Autodesk Inventor part; units mm, degrees
ref_plane "YZ Plane" through (0, 0, 0) normal (1, 0, 0) x (0, 1, 0)
ref_plane "XZ Plane" through (0, 0, 0) normal (0, 1, 0) x (-1, 0, 0)
ref_plane "XY Plane" through (0, 0, 0) normal (0, 0, 1) x (1, 0, 0)
sketch "Sketch1" plane through (0, 0, 0) normal (0, 1, 0) x (-1, 0, 0)
  line L0 (0, 0) -> (0, -167)
  circle A0 centre (0, 0) radius 1.7
  circle A1 centre (0, -167) radius 1.7
  circle A2 centre (0, 0) radius 2.5
  circle A3 centre (0, -167) radius 2.5
  line L1 (2.5, -167) -> (2.5, 0)
  line L2 (-2.5, 0) -> (-2.5, -167)
  dimension "d0" = 167
  dimension "d1" = 3.4
  dimension "d2" = 3.4
  dimension "d3" = 5
  dimension "d4" = 5
extrude "Extrusion1" add sketch "Sketch1" along normal blind 3
properties part number "HENK"
Check sheet for the modelled part. Datum: model origin and axes. Units: mm. Round coordinates to 2 decimals unless told otherwise and drop trailing zeros. Write each loop counter-clockwise with the first axis right and the second up, starting at its lowest first coordinate (ties: lowest second). Pieces come first, ordered by that corner, then holes. Notation, with made-up numbers: (-19, 43) -> (18, 43) arc R21 ccw to (18, 60) -> close; hole circle Ø11 at (-5.75, -19). An arc over 180 degrees is marked (long way). Answer as CSV lines item,"result". Start each with the question number.
1) Go/stop test with flat-tipped pins: P1, Ø1.5, axis at x = 1, y = 2, coming from the -Z side; P2, Ø2, axis at x = -1, z = -49, coming from the -Y side. Record where each tip stops, or that it passes through.
2) Material ranges on line 1 (Z direction, x = 0, y = 0.75); line 2 (X direction, y = 1.1, z = 0); line 3 (Z direction, x = 1.5, y = 1.3), recorded low to high. Write a range as from..to.
3) Release check for a two-part mould opening along Z. For faces 1 (the cylindrical face through (-0.1, 1.5, -169.5)), 2 (the cylindrical face through (0.37, 1.48, -165.34)), 3 (the flat face through (-2.5, 1, -85)), 4 (the cylindrical face through (0.1, 1.5, 2.5)) record: pulls with the +Z half, pulls with the -Z half, needs draft (parallel to the pull), parting line crosses it, or undercut.
4) Section check B-B on y = 2.1. Enter the section's corners in (x, z).
5) Section check A-A on x = 0. Enter the section's corners in (y, z).
Found:
1,P1,"stops at z = -169.49"
1,P2,"stops at y = 0"
2,line 1,"z = -169.5..-168.7, -165.3..-1.7, 1.7..2.5"
2,line 2,"x = -2.5..-1.7, 1.7..2.5"
2,line 3,"z = -169..-167.8, -166.2..-0.8, 0.8..2"
3,face 1,"pulls with the -Z half"
3,face 2,"undercut"
3,face 3,"needs draft"
3,face 4,"pulls with the +Z half"
4,outline,"(-2.5, -167) arc R2.5 ccw to (2.5, -167) -> (2.5, 0) arc R2.5 ccw to (-2.5, 0) -> close; hole circle Ø3.4 at (0, -167); hole circle Ø3.4 at (0, 0)"
5,outline,"(0, -169.5) -> (3, -169.5) -> (3, -168.7) -> (0, -168.7) -> close; (0, -165.3) -> (3, -165.3) -> (3, -1.7) -> (0, -1.7) -> close; (0, 1.7) -> (3, 1.7) -> (3, 2.5) -> (0, 2.5) -> close"
